from build123d import *

# Parameters (mm, degrees)
F0_R     = 25.4
F0_R_2   = 1.5875
F1_DEPTH = 25.4
F2_SIZE  = 2.54
F3_R     = 4.445


with BuildPart() as f1:
    # F0 (on Top) → F1 (new body)
    with BuildSketch(Plane.XY):
        Circle(F0_R)
        Circle(F0_R_2, mode=Mode.SUBTRACT)
    extrude(amount=F1_DEPTH)

    # F2
    f2_edges = [f1.edges().sort_by_distance(p)[0] for p in [
        (-25.4, 0, 25.4),
    ]]
    chamfer(f2_edges, length=F2_SIZE)

    # F3
    f3_edges = [f1.edges().sort_by_distance(p)[0] for p in [
        (-1.5875, 0, 25.4),
    ]]
    fillet(f3_edges, radius=F3_R)


solid = f1.part
Build history of the part. All positions in model axes, mm. Round coordinates to 2 decimals unless told otherwise and drop trailing zeros. Write each loop counter-clockwise with the first axis right and the second up, starting at its lowest first coordinate (ties: lowest second). Pieces come first, ordered by that corner, then holes. Notation, with made-up numbers: M -4,6 L 19,6 A17 ccw 19,24 Z; hole C 86.5,-33.5 d10. An arc over 180 degrees is marked long. Answer as a JSON object with one key per item and string values. Group by question number.
(1) Cut at C-C (z = 18.75). Give the cut face in (x, y) (1 decimal), and give its area (3 significant figures).
(2) Flat gauge pins, fed straight in: pin 1 (12 mm diameter, centred on y = 6.5, z = 17, fed in from +X); pin 2 (3 mm diameter, centred on y = 18, z = 12, fed in from -X); pin 3 (12 mm diameter, centred on y = -10, z = 9.5, fed in from -X). Where does each tip first touch, or does it go through?
(3) Mould opens along Y. For faces 1 (the conical face through (-4.982, -22.437, 25.277)), 2 (the flat face through (5, -5, 25.4)), 3 (the cylindrical face through (-0.34, -1.55, 10.33)) say: pulls with the +Y half, pulls with the -Y half, needs draft (parallel to the pull), parting line crosses it, or undercut.
(4) Cut at A-A (x = 0). Give the cut face in (y, z) (1 decimal), and give its area (3 significant figures).
(5) Drill centre lines: L1, parallel to Y at x = 0, z = 8; L2, parallel to X at y = 15, z = 7.75; L3, parallel to X at y = -5.5, z = 10. Where is each one in solid material? Low to high.
Responses:
{
 "1": {"outline": "C 0,0 d50.8; hole C 0,0 d3.2", "area": "2,020 mm2"},
 "2": {"pin 1": "stops at x = 25.4", "pin 2": "stops at x = -19.31", "pin 3": "stops at x = -25.08"},
 "3": {"face 1": "parting line crosses it", "face 2": "needs draft", "face 3": "undercut"},
 "4": {"outline": "M -25.4,0 L -1.6,0 L -1.6,21 A4.4 ccw -6,25.4 L -22.9,25.4 L -25.4,22.9 Z; M 1.6,0 L 25.4,0 L 25.4,22.9 L 22.9,25.4 L 6,25.4 A4.4 ccw 1.6,21 Z", "area": "1,190 mm2"},
 "5": {"L1": "y = -25.4 to -1.59, 1.59 to 25.4", "L2": "x = -20.5 to 20.5", "L3": "x = -24.8 to 24.8"}
}
